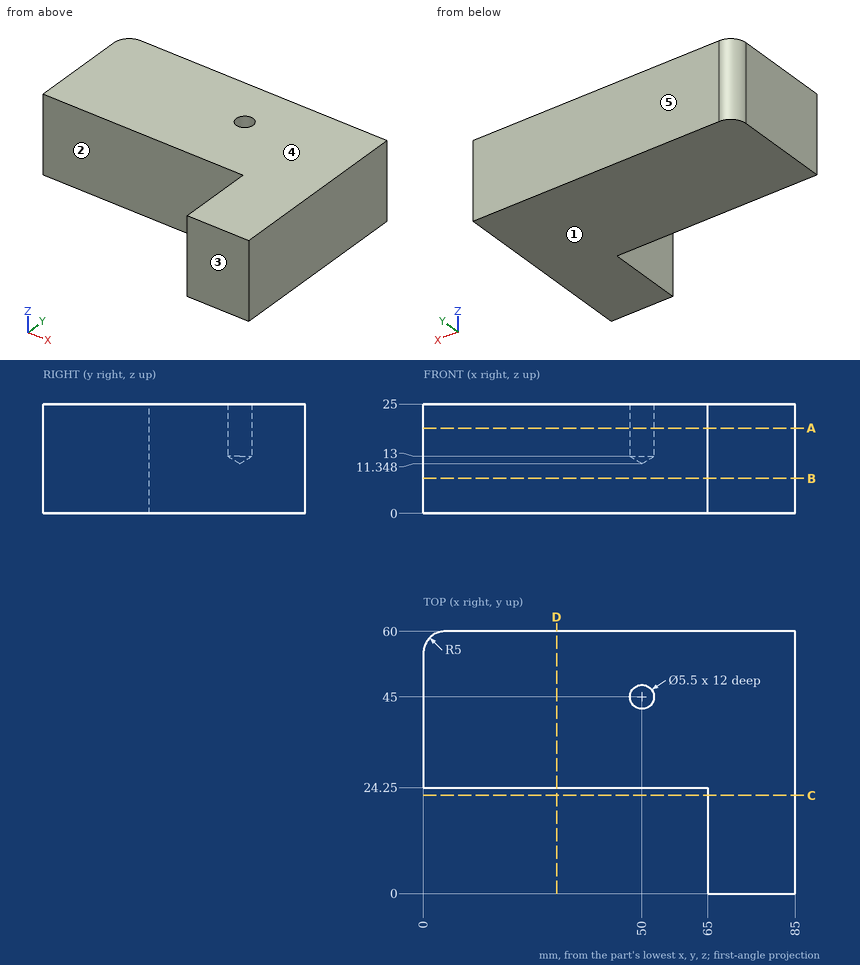
Verification items for this drawing (mm, ordinates from the low corner). A direction names the side the tool comes from. Give positions to 0.01 mm unless a question says otherwise; leave off trailing zeros. Loops run counter-clockwise (first coordinate to the right, second up) from the corner with the lowest first, then second, coordinate; pieces in that order, holes last. Notation, with made-up numbers: M 23.25,-6 L 56.25,-6 A18 cw 56.25,22 Z; hole C 33.5,71.25 d1. An arc over 180 degrees is marked long. Return JSON: item names as keys, results as strings. Group by question number.
1. Thickness scan on L1, parallel to X at y = 45, z = 16.5; L2, parallel to Y at x = 50, z = 17; L3, parallel to Y at x = 20.5, z = 15.5. Record the ranges inside material, lowest first.
2. Cross-section at B-B on z = 8. Record the boundary of the cut face in (x, y).
3. Cross-section at A-A on z = 19.5. Record the boundary of the cut face in (x, y).
4. Cross-section at D-D on x = 30.5. Record the boundary of the cut face in (y, z).
5. Mould release check, pull along Y, two halves, no side actions. Record for the marked faces 3, 4 and 5: released by +Y, released by -Y, zero draft, split by the parting line, or undercut.
6. Go/stop test with flat-tipped pins: pin 1 (8 mm diameter, centred on y = 7.5, z = 2.5, fed in from -X); pin 2 (3 mm diameter, centred on x = 40.5, z = 10.5, fed in from -Y). Record where each tip stops, or that it passes through.
7. Tool access check on the marked faces 1 and 2. Record the directions out of +Z, -Z, +X, -X, +Y, -Y that give a thin tool (end or side, any length) a straight path to the whole face; none if there is none.
8. Cross-section at C-C on y = 22.5. Record the boundary of the cut face in (x, z), plus the area to 3 significant figures.
Return value:
{
 "1": {"L1": "0 to 47.25, 52.75 to 85", "L2": "24.25 to 42.25, 47.75 to 60", "L3": "24.25 to 60"},
 "2": {"outline": "M 0,24.25 L 65,24.25 L 65,0 L 85,0 L 85,60 L 5,60 A5 ccw 0,55 Z"},
 "3": {"outline": "M 0,24.25 L 65,24.25 L 65,0 L 85,0 L 85,60 L 5,60 A5 ccw 0,55 Z; hole C 50,45 d5.5"},
 "4": {"outline": "M 24.25,0 L 60,0 L 60,25 L 24.25,25 Z"},
 "5": {"face 3": "released by -Y", "face 4": "zero draft", "face 5": "released by +Y"},
 "6": {"pin 1": "x = 65", "pin 2": "y = 24.25"},
 "7": {"face 1": "-Z, +X, -X, +Y, -Y", "face 2": "+Z, -Z, -X, -Y"},
 "8": {"outline": "M 65,0 L 85,0 L 85,25 L 65,25 Z", "area": "500 mm^2"}
}
